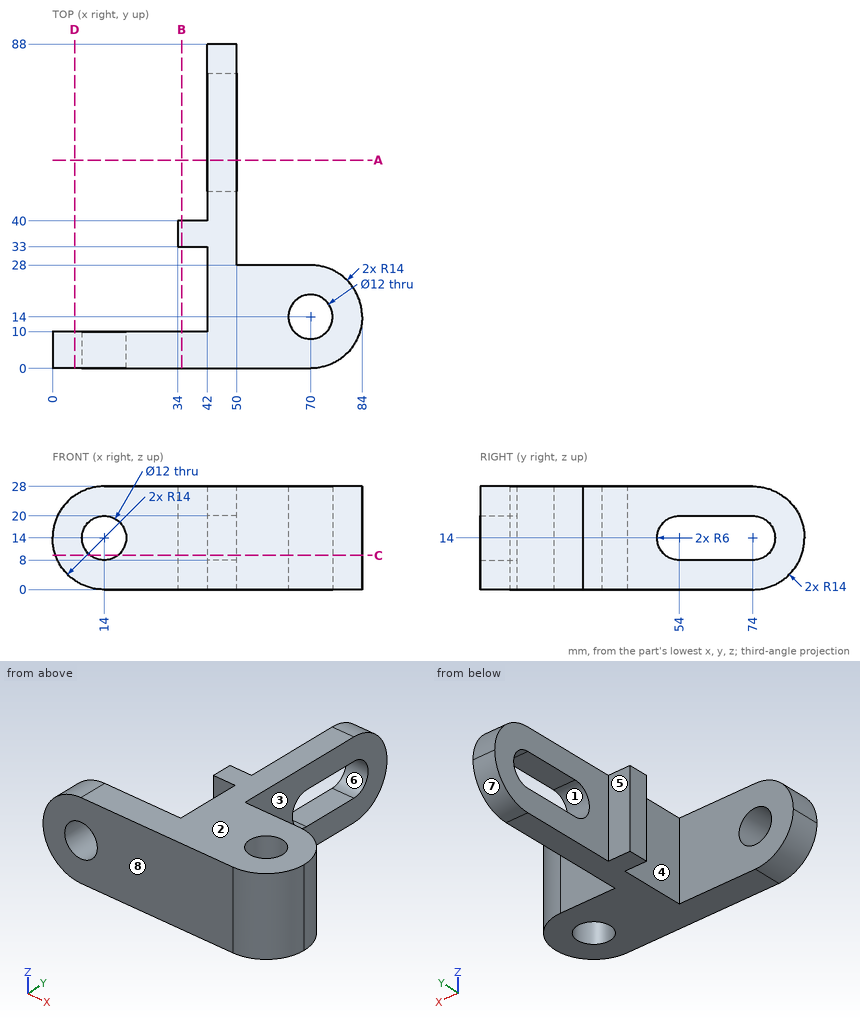
Job drawing, mm, ordinate dimensions from the low corner. One solid piece. A direction names the side the tool comes from. Coordinates: 2 decimals unless noted, no trailing zeros. Write each loop counter-clockwise with the first axis right and the second up, starting at its lowest first coordinate (ties: lowest second). Pieces come first, ordered by that corner, then holes. Notation, with made-up numbers: (78.5, -32.5) - (100.5, -32.5) arc R24 ccw to (100.5, -21.5) - close; hole circle Ø11 at (20.25, -28). An arc over 180 degrees is marked (long way). Use a Markdown table: item, result. Add a question column.
Item 1: Band-saw the part on C-C, the plane z = 9.25. Give the number of separate pieces and of enclosed holes in the cut face, and give its area (3 significant figures).
Item 2: 3-axis set-ups, long thin cutter, end or side, ignore diameter. For the marked faces 1, 2, 3, 4 and 5: which of +Z, -Z, +X, -X, +Y, -Y reach the whole face in a straight line?
Item 3: Band-saw the part on A-A, the plane y = 56.5. Give the cut face in (x, z), and give its area (3 significant figures).
Item 4: Mould opens along Z. For the marked faces 6, 7 and 8 say: pulls with the +Z half, pulls with the -Z half, needs draft (parallel to the pull), parting line crosses it, or undercut.
Item 5: Band-saw the part on D-D, the plane x = 6. Give the cut face in (y, z), and give its area (3 significant figures).
Item 6: Band-saw the part on B-B, the plane x = 35. Give the cut face in (y, z), and give its area (3 significant figures).
Item 7: Drill centre lines: L1, parallel to Y at x = 70, z = 13.5; L2, parallel to Y at x = 36.5, z = 7.75. Where is each one in solid material? Low to high. Write a range as from..to.
Item 8: Flat gauge pins, fed straight in: pin 1 (3 mm diameter, centred on y = 38, z = 5.5, fed in from +X); pin 2 (19 mm diameter, centred on x = 70, y = 14, fed in from -Z); pin 3 (8 mm diameter, centred on x = 22.5, z = 8.5, fed in from +Y); pin 4 (1 mm diameter, centred on x = 71.5, z = 7, fed in from -Y). Where does each tip first touch, or does it go through?
Numbers:
| question | item | result |
|---|---|---|
| 1 | separate pieces | 3 |
| 1 | enclosed holes | 1 |
| 1 | area | 1,630 mm2 |
| 2 | face 1 | +X, -X |
| 2 | face 2 | +Z, +X, -X, +Y, -Y |
| 2 | face 3 | +Z, -Z, +X, +Y |
| 2 | face 4 | +Z, -Z, -X |
| 2 | face 5 | +Z, -Z, -X, +Y |
| 3 | outline | (42, 0) - (50, 0) - (50, 8) - (42, 8) - close; (42, 20) - (50, 20) - (50, 28) - (42, 28) - close |
| 3 | area | 128 mm2 |
| 4 | face 6 | undercut |
| 4 | face 7 | pulls with the -Z half |
| 4 | face 8 | needs draft |
| 5 | outline | (0, 2.51) - (10, 2.51) - (10, 25.49) - (0, 25.49) - close |
| 5 | area | 230 mm2 |
| 6 | outline | (0, 0) - (10, 0) - (10, 28) - (0, 28) - close; (33, 0) - (40, 0) - (40, 28) - (33, 28) - close |
| 6 | area | 476 mm2 |
| 7 | L1 | 0..8, 20..28 |
| 7 | L2 | 0..10, 33..40 |
| 8 | pin 1 | x = 50 |
| 8 | pin 2 | z = 0 |
| 8 | pin 3 | y = 10 |
| 8 | pin 4 | y = 0.04 |
